Design review of the part built by this model. Coordinates are the model's own, in mm. Face numbers are marked on the shaded views. A direction names the side the tool comes from. Round coordinates to 2 decimals unless told otherwise and drop trailing zeros. Loops run counter-clockwise (first coordinate to the right, second up) from the corner with the lowest first, then second, coordinate; pieces in that order, holes last. Notation, with made-up numbers: (-9, 79.25) - (0, 79.25) arc R13 ccw to (0, 97.25) - close; hole circle Ø11 at (13, -6). An arc over 180 degrees is marked (long way). Return JSON: item names as keys, results as strings. Group by question number.
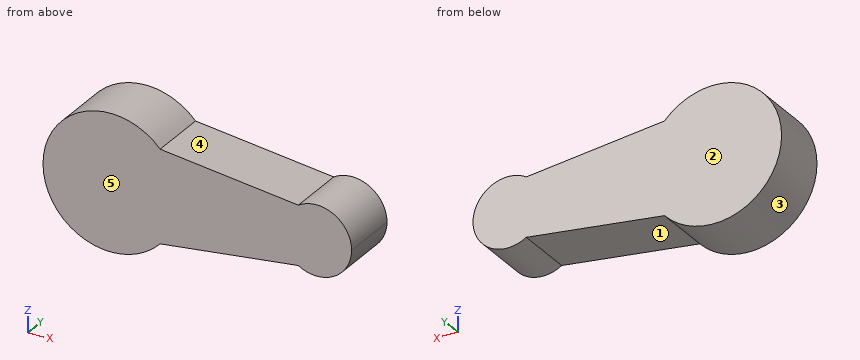
from build123d import *

# Parameters (mm, degrees)
F1_DEPTH = 12.7


with BuildPart() as f1:
    # F0 (on Front) → F1 (new body, symmetric)
    with BuildSketch(Plane.XZ):
        with BuildLine():
            ThreePointArc((-18.237302, -19.674743), (-12.488315, -10.574656), (-10.47857, 0))
            ThreePointArc((-10.47857, 0), (-12.488315, 10.574656), (-18.237302, 19.674743))
            ThreePointArc((-18.237302, 19.674743), (-68.128892, 0), (-18.237302, -19.674743))
        make_face()
        with BuildLine():
            ThreePointArc((-18.237302, 19.674743), (-12.488315, 10.574656), (-10.47857, 0))
            ThreePointArc((-10.47857, 0), (-12.488315, -10.574656), (-18.237302, -19.674743))
            Line((-18.237302, -19.674743), (40.605832, -12.550029))
            ThreePointArc((40.605832, -12.550029), (33.664157, 0), (40.605832, 12.550029))
            Line((40.605832, 12.550029), (-18.237302, 19.674743))
        make_face()
        with BuildLine():
            ThreePointArc((63.295345, 0), (55.650701, 12.96454), (40.605832, 12.550029))
            ThreePointArc((40.605832, 12.550029), (33.664157, 0), (40.605832, -12.550029))
            ThreePointArc((40.605832, -12.550029), (55.650701, -12.96454), (63.295345, 0))
        make_face()
    extrude(amount=F1_DEPTH, both=True)


solid = f1.part
Q1. For line 1 (Z direction, x = -50, y = -10.5); line 2 (X direction, y = 0.75, z = 26.5); line 3 (Z direction, x = -12, y = 8.25), list the stretches that pass through material, from the lowest coordinate up.
Q2. Add section B-B, the plane x = 15. State the section outline as (y, z) points.
Q3. Add section A-A, the plane y = -8.75. State the section outline as (x, z) points, plus the area to 3 significant figures.
Q4. Draft analysis for pull direction X (two halves, no side actions). For the marked faces 1, 2 and 3, state which applies: pulls with the +X half, pulls with the -X half, needs draft (parallel to the pull), parting line crosses it, or undercut.
Q5. Insertion check: pin 1 Ø5 at (y, z) = (2.5, 21.5) entering from -X; pin 2 Ø12 at (x, y) = (-24.5, -5.5) entering from -Z; pin 3 Ø4 at (x, y) = (-33.5, 10) entering from +Z. Each pin has a flat end and moves straight along its axis. Give the tip position at first contact, or say it passes through.
Q6. Tool access review of the marked faces 4 and 5: name each direction out of +Z, -Z, +X, -X, +Y, -Y from which nothing blocks a thin tool from reaching the whole face with its end or side.
Q7. Add section C-C, the plane z = -10.5. State the section outline as (x, y) points.
Evaluation:
{
 "1": {"line 1": "-26.77 to 26.77", "line 2": "-50.65 to -27.96", "line 3": "-18.92 to 18.92"},
 "2": {"outline": "(-12.7, -15.65) - (12.7, -15.65) - (12.7, 15.65) - (-12.7, 15.65) - close"},
 "3": {"outline": "(-18.24, -19.67) - (40.61, -12.55) arc R14.82 ccw (long way) to (40.61, 12.55) - (-18.24, 19.67) arc R28.83 ccw (long way) to start", "area": "4,860 mm²"},
 "4": {"face 1": "undercut", "face 2": "needs draft", "face 3": "parting line crosses it"},
 "5": {"pin 1": "x = -60.98", "pin 2": "z = -27.45", "pin 3": "z = 28.57"},
 "6": {"face 4": "+Z, +Y, -Y", "face 5": "+Z, -Z, +X, -X, -Y"},
 "7": {"outline": "(-66.15, -12.7) - (58.93, -12.7) - (58.93, 12.7) - (-66.15, 12.7) - close"}
}
